from build123d import *

# Parameters (mm, degrees)
PAD_DEPTH       = 10.1
POCKET_DEPTH    = 1.5
POCKET001_DEPTH = 1.5
FILLET003_R     = 1


with BuildPart() as part:
    # Sketch → Pad (new body)
    with BuildSketch(Plane.XY):
        with BuildLine():
            ThreePointArc((-4.411122, 6.35), (-10.761122, 0), (-4.411122, -6.35))
            Line((14.538878, -6.35), (-4.411122, -6.35))
            Line((14.538878, 6.35), (14.538878, -6.35))
            Line((-4.411122, 6.35), (14.538878, 6.35))
        make_face()
    extrude(amount=PAD_DEPTH)

    # Sketch003 → Pocket (cut)
    with BuildSketch(Plane.XY):
        with BuildLine():
            ThreePointArc((12.288878, 2.25), (10.038878, 0), (12.288878, -2.25))
            Line((12.288878, -2.25), (14.538878, -2.25))
            Line((14.538878, 2.25), (14.538878, -2.25))
            Line((12.288878, 2.25), (14.538878, 2.25))
        make_face()
    extrude(amount=POCKET_DEPTH, mode=Mode.SUBTRACT)

    # Sketch004 → Pocket001 (cut)
    with BuildSketch(Plane.XY):
        with BuildLine():
            ThreePointArc((-8.632006, -2.25), (-6.382006, 0), (-8.632006, 2.25))
            Line((-8.632006, 2.25), (-10.882006, 2.25))
            Line((-10.882006, 2.25), (-10.882006, -2.25))
            Line((-10.882006, -2.25), (-8.632006, -2.25))
        make_face()
    extrude(amount=POCKET001_DEPTH, mode=Mode.SUBTRACT)

    # Fillet003
    fillet003_edges = [part.edges().sort_by_distance(p)[0] for p in [
        (14.538878, -6.35, 5.05),
        (14.538878, 6.35, 5.05),
        (5.063878, -6.35, 0),
        (14.538878, -4.3, 0),
        (14.538878, 4.3, 0),
        (5.063878, 6.35, 0),
        (-8.019099, 5.225419, 0),
        (-8.019099, -5.225419, 0),
    ]]
    fillet(fillet003_edges, radius=FILLET003_R)


solid = part.part
Work out the finished part from the listing and answer in its coordinate system (mm). A direction names the side the tool comes from. Give positions to 0.01 mm unless a question says otherwise; leave off trailing zeros. Loops run counter-clockwise (first coordinate to the right, second up) from the corner with the lowest first, then second, coordinate; pieces in that order, holes last. Notation, with made-up numbers: (-7, 2.5) - (46, 2.5) arc R5 cw to (46, 10.5) - close; hole circle Ø3 at (60.5, -23.75). An arc over 180 degrees is marked (long way). Answer in a Markdown table with one row per item.
(1) Section C-C (y = 1.5) is taken. Give the vertices of the cut face in (x, z).
Results list:
| item | result |
|---|---|
| outline | (-10.58, 1.5) - (-6.95, 1.5) - (-6.95, 0) - (10.61, 0) - (10.61, 1.5) - (14.54, 1.5) - (14.54, 10.1) - (-10.58, 10.1) - close |
(2) Section A-A (y = 0) is taken. Give the vertices of the cut face in (x, z), and give its area (3 significant figures).
Results list:
| item | result |
|---|---|
| outline | (-10.76, 1.5) - (-6.38, 1.5) - (-6.38, 0) - (10.04, 0) - (10.04, 1.5) - (14.54, 1.5) - (14.54, 10.1) - (-10.76, 10.1) - close |
| area | 242 mm² |
(3) Consider L1, parallel to X at y = -0.25, z = 4.5; L2, parallel to X at y = 2.25, z = 2.5; L3, parallel to Y at x = 13.25, z = 0.5. Determine where each line is inside the solid, lowest interval first. Write a range as [from, to].
Results list:
| item | result |
|---|---|
| L1 | x = [-10.76, 14.54] |
| L2 | x = [-10.35, 14.54] |
| L3 | y = [-6.22, -2.25], [2.25, 6.22] |
(4) For a pull along Y with two mould halves and no side action, classify faces 1 (the face through (-10.76, 0.14, 5.49)), 2 (the face through (12, 0, 1.5)), 3 (the face through (2, 0, 0)) as pulls with the +Y half, pulls with the -Y half, needs draft (parallel to the pull), parting line crosses it, or undercut.
Results list:
| item | result |
|---|---|
| face 1 | parting line crosses it |
| face 2 | undercut |
| face 3 | needs draft |
(5) A tool of negligible diameter and unlimited length cuts with its end or side. For faces 4 (the face through (13, 2.25, 1)), 5 (the face through (14.2, 6.1, 5.6)), 6 (the face through (-9, 0, 1.5)), from which of +Z, -Z, +X, -X, +Y, -Y can it reach the whole face along a straight path? Write none if from no direction.
Results list:
| item | result |
|---|---|
| face 4 | -Z, +X |
| face 5 | +Z, -Z, +X, +Y |
| face 6 | -Z, -X |
(6) Flat-ended cylindrical pins translate along their axes: pin 1 Ø3 at (x, z) = (-6.5, 6.5) entering from -Y; pin 2 Ø1 at (y, z) = (-1, 7.5) entering from -X; pin 3 Ø0.8 at (x, z) = (-9, 1) entering from +Y. Find the tip coordinate at first contact, or state that the pin passes through.
Results list:
| item | result |
|---|---|
| pin 1 | stops at y = -6.32 |
| pin 2 | stops at x = -10.74 |
| pin 3 | stops at y = 4.77 |
(7) Section B-B (z = 5.25) is taken. Give the vertices of the cut face in (x, y), and give its area (3 significant figures).
Results list:
| item | result |
|---|---|
| outline | (-4.41, -6.35) - (13.54, -6.35) arc R1 ccw to (14.54, -5.35) - (14.54, 5.35) arc R1 ccw to (13.54, 6.35) - (-4.41, 6.35) arc R6.35 ccw to start |
| area | 304 mm² |
